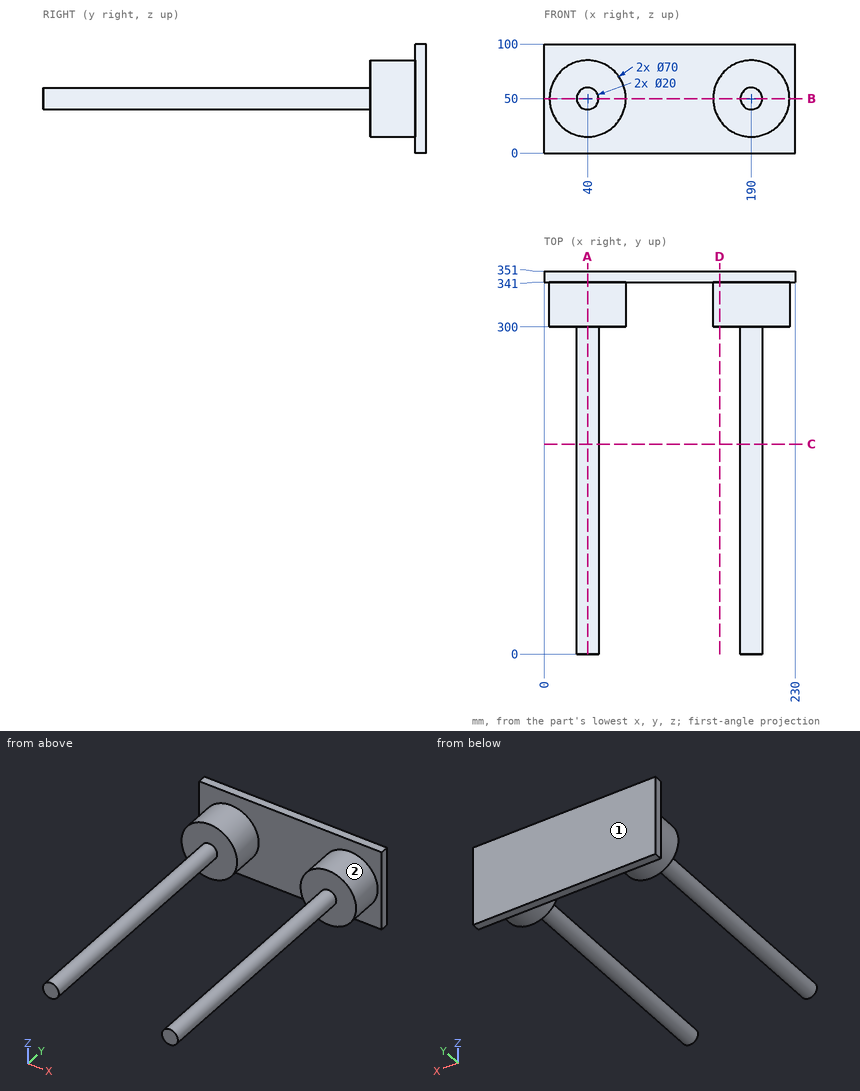
Drawing for the job (mm, zero at the part's lowest x, y, z). Round coordinates to 2 decimals unless told otherwise and drop trailing zeros. Write each loop counter-clockwise with the first axis right and the second up, starting at its lowest first coordinate (ties: lowest second). Pieces come first, ordered by that corner, then holes. Notation, with made-up numbers: M 3.5,39.5 L 59.5,39.5 A20 cw 59.5,46.5 Z; hole C -25.75,69.25 d9. An arc over 180 degrees is marked long. Answer as a JSON object with one key per item and string values. Group by question number.
(1) Cut at A-A (x = 40). Give the cut face in (y, z).
(2) Flat gauge pin, fed straight in: pin 1 (10 mm diameter, centred on x = 191, y = 189, fed in from -Z). Where does the tip first touch, or does it go through?
(3) Mould opens along X. For the marked faces 1 and 2 say: pulls with the +X half, pulls with the -X half, needs draft (parallel to the pull), parting line crosses it, or undercut.
(4) Cut at C-C (y = 192.5). Give the cut face in (x, z).
(5) Cut at B-B (z = 50). Give the cut face in (x, y), and give its area (3 significant figures).
(6) Cut at D-D (x = 161). Give the cut face in (y, z), and give its area (3 significant figures).
(7) Drill centre lines: L1, parallel to X at y = 333, z = 49.5; L2, parallel to X at y = 70.5, z = 50.5; L3, parallel to Y at x = 144.5, z = 83. Where is each one in solid material? Low to high.
Responses:
{
 "1": {"outline": "M 0,40 L 300,40 L 300,15 L 341,15 L 341,0 L 351,0 L 351,100 L 341,100 L 341,85 L 300,85 L 300,60 L 0,60 Z"},
 "2": {"pin 1": "stops at z = 40"},
 "3": {"face 1": "needs draft", "face 2": "undercut"},
 "4": {"outline": "C 40,50 d20; C 190,50 d20"},
 "5": {"outline": "M 0,341 L 5,341 L 5,300 L 30,300 L 30,0 L 50,0 L 50,300 L 75,300 L 75,341 L 155,341 L 155,300 L 180,300 L 180,0 L 200,0 L 200,300 L 225,300 L 225,341 L 230,341 L 230,351 L 0,351 Z", "area": "20,000 mm2"},
 "6": {"outline": "M 300,30.4 L 341,30.4 L 341,0 L 351,0 L 351,100 L 341,100 L 341,69.6 L 300,69.6 Z", "area": "2,610 mm2"},
 "7": {"L1": "x = 5 to 75, 155 to 225", "L2": "x = 30.01 to 49.99, 180.01 to 199.99", "L3": "y = 341 to 351"}
}
